Verification items for the finished model (mm, model axes). Round coordinates to 2 decimals unless told otherwise and drop trailing zeros. Order: outer loops, then holes, each group sorted by start corner. A loop starts at its lowest first (then second) coordinate and runs counter-clockwise, first axis right, second up. Notation, with made-up numbers: (-37.5, 87) -> (6.5, 87) arc R19 cw to (6.5, 118) -> close; hole circle Ø10 at (-36, -1). An arc over 180 degrees is marked (long way). Return JSON: item names as keys, results as strings. Group by question number.
Item 1: Sectioned sample at A-A on x = -120. Record the cut outline in (y, z).
Item 2: Draft check along X on faces 1 (the cylindrical face through (-163.966, 0.521, -0.14)), 2 (the flat face through (3, -100, 0)), 3 (the flat face through (200, 1, 0)), 4 (the flat face through (-200, -1, 0)). Enter one of: pulls with the +X half, pulls with the -X half, needs draft (parallel to the pull), parting line crosses it, or undercut.
Item 3: Depth check by flat-ended pin: pin 1 Ø6.5 at (x, y) = (190, 40) entering from +Z. Enter the tip coordinate at first touch or a pass-through.
Item 4: Scan lines: probe 1 along X at (y, z) = (0, 0.75); probe 2 along Y at (x, z) = (190, 2); probe 3 along Y at (x, z) = (60, 6.25). Record each from-to range of solid material in increasing order. Write a range as from..to.
Item 5: Sectioned sample at C-C on x = 190. Record the cut outline in (y, z), plus the area to 3 significant figures.
Item 6: Sectioned sample at B-B on y = 80. Record the cut outline in (x, z).
Autodesk Inventor part; units mm, degrees
ref_plane "YZ Plane" through (0, 0, 0) normal (1, 0, 0) x (0, 1, 0)
ref_plane "XZ Plane" through (0, 0, 0) normal (0, 1, 0) x (-1, 0, 0)
ref_plane "XY Plane" through (0, 0, 0) normal (0, 0, 1) x (1, 0, 0)
sketch "Sketch1" plane through (0, 0, 0) normal (0, 0, 1) x (1, 0, 0)
  line L0 (-200, 100) -> (200, 100)
  line L1 (200, 100) -> (200, -100)
  line L2 (200, -100) -> (-200, -100)
  line L3 (-200, -100) -> (-200, 100)
  point P0 (0, 0)
  point P1 (0, 100)
  point P2 (-200, 0)
  dimension "d0" = 400
  dimension "d1" = 200
extrude "Extrusion1" add sketch "Sketch1" along normal mid plane 20
sketch "Sketch10" plane through (0, 0, 10) normal (0, 0, 1) x (1, 0, 0)
  line L0 (-200, 100) -> (-200, -100)
  point P0 (0, 0)
  point P1 (-160, 0)
  dimension "d53" = 40
hole "Hole1" at (-160, 0, 10) direction (0, 0, -1) diameter 8 end through all
pattern_linear "Rectangular Pattern1" count 2 spacing 40 along (1, 0, 0) count 2 spacing 180 along (1, 0, 0) of "Hole1"
sketch "Sketch11" plane through (0, 0, 10) normal (0, 0, 1) x (1, 0, 0)
  line L0 (200, -100) -> (200, 100)
  point P0 (0, 0)
  point P1 (190, 0)
  point P2 (200, 0)
  dimension "d57" = 10
hole "Hole2" at (190, 0, 10) direction (0, 0, -1) diameter 8 end through all
pattern_linear "Rectangular Pattern2" count 5 spacing 40 along (0, 1, 0) of "Hole2" first direction both ways yes
properties part number "0005-10-024" material "Wood (Maple)"
Recorded:
{
 "1": {"outline": "(-100, -10) -> (-4, -10) -> (-4, 10) -> (-100, 10) -> close; (4, -10) -> (100, -10) -> (100, 10) -> (4, 10) -> close"},
 "2": {"face 1": "undercut", "face 2": "needs draft", "face 3": "pulls with the +X half", "face 4": "pulls with the -X half"},
 "3": {"pin 1": "through"},
 "4": {"probe 1": "-200..-164, -156..-124, -116..16, 24..56, 64..186, 194..200", "probe 2": "-100..-84, -76..-44, -36..-4, 4..36, 44..76, 84..100", "probe 3": "-100..-4, 4..100"},
 "5": {"outline": "(-100, -10) -> (-84, -10) -> (-84, 10) -> (-100, 10) -> close; (-76, -10) -> (-44, -10) -> (-44, 10) -> (-76, 10) -> close; (-36, -10) -> (-4, -10) -> (-4, 10) -> (-36, 10) -> close; (4, -10) -> (36, -10) -> (36, 10) -> (4, 10) -> close; (44, -10) -> (76, -10) -> (76, 10) -> (44, 10) -> close; (84, -10) -> (100, -10) -> (100, 10) -> (84, 10) -> close", "area": "3,200 mm²"},
 "6": {"outline": "(-200, -10) -> (186, -10) -> (186, 10) -> (-200, 10) -> close; (194, -10) -> (200, -10) -> (200, 10) -> (194, 10) -> close"}
}
